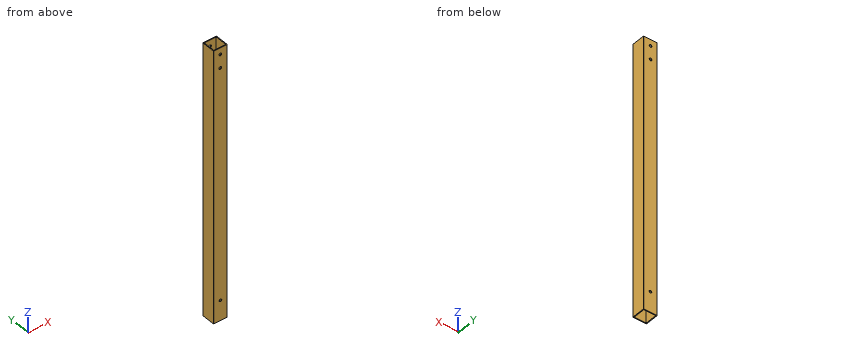
```python
from build123d import *

# Parameters (mm, degrees)
SKETCH1_W           = 22.225
SKETCH1_H           = 22.225
BOSS_EXTRUDE1_DEPTH = 508
SKETCH7_R           = 2.54
CUT_EXTRUDE5_DEPTH  = 26.4
SKETCH8_R           = 2.4892
CUT_EXTRUDE6_DEPTH  = 25.4


with BuildPart() as part:
    # Sketch1 → Boss-Extrude1 (new body)
    with BuildSketch(Plane(origin=(0, 0, 0), x_dir=(-1, 0, 0), z_dir=(0, 0, -1))):
        with BuildLine():
            Line((1.5875, -1.3335), (1.5875, 23.5585))
            ThreePointArc((1.5875, 23.5585), (1.513105122, 23.738105122), (1.3335, 23.8125))
            Line((1.3335, 23.8125), (-23.5585, 23.8125))
            ThreePointArc((-23.5585, 23.8125), (-23.738105122, 23.738105122), (-23.8125, 23.5585))
            Line((-23.8125, 23.5585), (-23.8125, -1.3335))
            ThreePointArc((-23.8125, -1.3335), (-23.738105122, -1.513105122), (-23.5585, -1.5875))
            Line((-23.5585, -1.5875), (1.3335, -1.5875))
            ThreePointArc((1.3335, -1.5875), (1.513105122, -1.513105122), (1.5875, -1.3335))
        make_face()
        with Locations((-11.1125, 11.1125)):
            Rectangle(SKETCH1_W, SKETCH1_H, mode=Mode.SUBTRACT)
    extrude(amount=-BOSS_EXTRUDE1_DEPTH)

    # Sketch7 → Cut-Extrude5 (cut, through all)
    with BuildSketch(Plane.XZ.offset(1.5875)):
        with Locations((10.9125, 470.65)):
            Circle(SKETCH7_R)
        with Locations((10.9125, 496.05)):
            Circle(SKETCH7_R)
    extrude(amount=-CUT_EXTRUDE5_DEPTH, mode=Mode.SUBTRACT)

    # Sketch8 → Cut-Extrude6 (cut)
    with BuildSketch(Plane(origin=(0, 23.8125, 0), x_dir=(1, 0, 0), z_dir=(0, 1, 0))):
        with Locations((11.1125, -37.933268304)):
            Circle(SKETCH8_R)
    extrude(amount=-CUT_EXTRUDE6_DEPTH, mode=Mode.SUBTRACT)


solid = part.part
```
Work out the finished part from the listing and answer in its coordinate system (mm). Give positions to 0.01 mm unless a question says otherwise; leave off trailing zeros. Order: outer loops, then holes, each group sorted by start corner. A loop starts at its lowest first (then second) coordinate and runs counter-clockwise, first axis right, second up. Notation, with made-up numbers: M 42.5,46.25 L 95.5,46.25 A27 cw 95.5,64.25 Z; hole C 46,87.5 d11. An arc over 180 degrees is marked long. Return JSON: item names as keys, results as strings.
1) Section A-A, the plane y = 15.75 is taken. Write down the section's boundary in (x, z) (1 decimal).
Resolved:
{"outline": "M -1.6,0 L 0,0 L 0,508 L -1.6,508 Z; M 22.2,0 L 23.8,0 L 23.8,508 L 22.2,508 Z"}
2) Straight lines are drawn through the part: line 1 along Y through (x, z) = (3.25, 161.5) (1 decimal); line 2 along X through (y, z) = (-0.75, 470.65). For each, find the intervals that lie inside material, in ascending order. Write a range as [from, to].
Resolved:
{"line 1": "[-1.6, 0], [22.2, 23.8]", "line 2": "[-1.59, 8.37], [13.45, 23.81]"}
3) This flat-tipped pin is pushed along its axis until it touches: pin 1 (6 mm diameter, centred on x = 10.91, z = 496.05, fed in from -Y). Where does it stop, or does it pass through?
Resolved:
{"pin 1": "y = -1.59"}
